For this review, take the finished solid that the model builds, in its own axes (mm). Face numbers are marked on the shaded views. A direction names the side the tool comes from. Give positions to 0.01 mm unless a question says otherwise; leave off trailing zeros. Order: outer loops, then holes, each group sorted by start corner. A loop starts at its lowest first (then second) coordinate and runs counter-clockwise, first axis right, second up. Notation, with made-up numbers: M 21,12 L 55,12 A16 cw 55,41 Z; hole C 7.5,22.25 d8. An arc over 180 degrees is marked long. Answer as CSV lines item,"result". Start each with the question number.
1. Clearance check with flat-ended pins moving along their axes: P1, Ø1.5, axis at x = -17.5, z = 0.5, coming from the +Y side; P2, Ø2.5, axis at x = -13.5, z = -18, coming from the -Y side; P3, Ø2.5, axis at y = 2.5, z = -16.5, coming from the -X side. State where each tip first meets the part, or that it passes through.
2. We need section B-B, the plane x = 0. Give the boundary of the cut face in (y, z), and give its area (3 significant figures).
3. Mouldability with a two-part tool opening along X and no side actions: class the marked faces 6, 7, 8 and 9 as pulls with the +X half, pulls with the -X half, needs draft (parallel to the pull), parting line crosses it, or undercut.
4. For line 1 along Z through (x, y) = (30, 14.25); line 2 along X through (y, z) = (6.75, -7.5); line 3 along X through (y, z) = (14.5, 16.5), list the stretches that pass through material, from the lowest coordinate up.
5. Machinability: for the marked faces 1, 2, 3, 4 and 5, which of the approach directions +Z, -Z, +X, -X, +Y, -Y give a long, thin tool a straight path to every point of the face, cutting with its end or side? Answer none if there is none.
6. We need section C-C, the plane z = 7.5. Give the boundary of the cut face in (x, y).
7. We need section A-A, the plane y = 15.5. State how many separate pieces and enclosed holes the cut face has, and give its area (3 significant figures).
8. We need section D-D, the plane x = 24. Give the boundary of the cut face in (y, z), and give its area (3 significant figures).
from build123d import *

# Parameters (mm, degrees)
SKETCH1_W                = 90
SKETCH1_H                = 30
BOSS_EXTRUDE1_DEPTH      = 7.5
SKETCH2_W                = 70
SKETCH2_H                = 30
BOSS_EXTRUDE2_DEPTH      = 10
CUT_EXTRUDE1_DEPTH       = 31
BOSS_EXTRUDE3_DEPTH      = 5
BOSS_EXTRUDE3_DEPTH_BACK = 35
CUT_EXTRUDE2_DEPTH       = 30
SKETCH7_R                = 2.25
CUT_EXTRUDE3_DEPTH       = 15


with BuildPart() as part:
    # Sketch1 → Boss-Extrude1 (new body, symmetric)
    with BuildSketch(Plane(origin=(0, 0, 0), x_dir=(1, 0, 0), z_dir=(0, 1, 0))):
        Rectangle(SKETCH1_W, SKETCH1_H)
    extrude(amount=BOSS_EXTRUDE1_DEPTH, both=True)

    # Sketch2 → Boss-Extrude2 (add)
    with BuildSketch(Plane(origin=(0, 7.5, 0), x_dir=(1, 0, 0), z_dir=(0, 1, 0))):
        Rectangle(SKETCH2_W, SKETCH2_H)
    extrude(amount=BOSS_EXTRUDE2_DEPTH)

    # Sketch3 → Cut-Extrude1 (cut, through all)
    with BuildSketch(Plane.XY.offset(15)):
        Polygon((-26.286782916, -2.5), (26.286782916, -2.5), (22.5, -7.5), (-22.5, -7.5), align=None)
    extrude(amount=-CUT_EXTRUDE1_DEPTH, mode=Mode.SUBTRACT)

    # Sketch4 → Boss-Extrude3 (add, two sides)
    with BuildSketch(Plane.XY.offset(15)) as boss_extrude3_sk:
        with BuildLine():
            Line((-7.5, 5), (-7.5, -2.5))
            Line((-7.5, -2.5), (7.5, -2.5))
            Line((7.5, -2.5), (7.5, 5))
            Line((7.5, 5), (17.5, 5))
            ThreePointArc((17.5, 5), (26.338834765, 8.661165235), (30, 17.5))
            Line((30, 17.5), (25, 17.5))
            ThreePointArc((25, 17.5), (17.5, 10), (10, 17.5))
            Line((10, 17.5), (-10, 17.5))
            ThreePointArc((-10, 17.5), (-17.5, 10), (-25, 17.5))
            Line((-25, 17.5), (-30, 17.5))
            ThreePointArc((-30, 17.5), (-26.338834765, 8.661165235), (-17.5, 5))
            Line((-17.5, 5), (-7.5, 5))
        make_face()
    extrude(amount=BOSS_EXTRUDE3_DEPTH)
    extrude(boss_extrude3_sk.sketch, amount=-BOSS_EXTRUDE3_DEPTH_BACK)

    # Sketch6 → Cut-Extrude2 (cut)
    with BuildSketch(Plane.XY.offset(15)):
        with BuildLine():
            Line((-25, 17.5), (-10, 17.5))
            ThreePointArc((-10, 17.5), (-17.5, 10), (-25, 17.5))
        make_face()
        with BuildLine():
            Line((10, 17.5), (25, 17.5))
            ThreePointArc((25, 17.5), (17.5, 10), (10, 17.5))
        make_face()
    extrude(amount=-CUT_EXTRUDE2_DEPTH, mode=Mode.SUBTRACT)

    # Sketch7 → Cut-Extrude3 (cut)
    with BuildSketch(Plane(origin=(0, 17.5, 0), x_dir=(1, 0, 0), z_dir=(0, 1, 0))):
        with Locations((0, 15)):
            Circle(SKETCH7_R)
        with Locations((0, -15)):
            Circle(SKETCH7_R)
        with Locations((-30, 7.5)):
            Circle(SKETCH7_R)
        with Locations((-30, -7.5)):
            Circle(SKETCH7_R)
        with Locations((30, -7.5)):
            Circle(SKETCH7_R)
        with Locations((30, 7.5)):
            Circle(SKETCH7_R)
    extrude(amount=-CUT_EXTRUDE3_DEPTH, mode=Mode.SUBTRACT)


solid = part.part
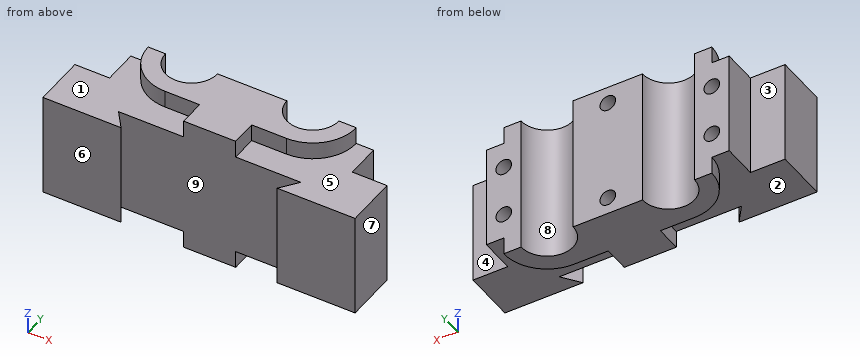
Result set:
1,P1,"y = 10.04"
1,P2,"y = 5"
1,P3,"x = -7.5"
2,outline,"M -2.5,-20 L 17.5,-20 L 17.5,-17.25 L 2.5,-17.25 L 2.5,-12.75 L 17.5,-12.75 L 17.5,12.75 L 2.5,12.75 L 2.5,17.25 L 17.5,17.25 L 17.5,20 L -2.5,20 Z"
2,area,"665 mm2"
3,face 6,"needs draft"
3,face 7,"pulls with the +X half"
3,face 8,"undercut"
3,face 9,"undercut"
4,line 1,"-15 to -9.75, -5.25 to 5.25, 9.75 to 15"
4,line 2,"-45 to -32.25, -27.75 to 27.75, 32.25 to 45"
4,line 3,"-29.63 to -24.37, -10.63 to -1.68, 1.68 to 10.63, 24.37 to 29.63"
5,face 1,"+Z, -X, -Y"
5,face 2,"-Z, -X, -Y"
5,face 3,"+Z, -Z, -X, +Y"
5,face 4,"+Z, -Z, +X, +Y"
5,face 5,"+Z, +X, -Y"
6,outline,"M -45,-7.5 L -22.5,-7.5 L -26.29,-2.5 L 26.29,-2.5 L 22.5,-7.5 L 45,-7.5 L 45,7.5 L 35,7.5 L 35,17.5 L 32.25,17.5 L 32.25,2.5 L 27.75,2.5 L 27.75,17.5 L 25,17.5 A7.5 cw 10,17.5 L -10,17.5 A7.5 cw -25,17.5 L -27.75,17.5 L -27.75,2.5 L -32.25,2.5 L -32.25,17.5 L -35,17.5 L -35,7.5 L -45,7.5 Z"
7,separate pieces,"3"
7,enclosed holes,"6"
7,area,"1,440 mm2"
8,outline,"M -7.5,-15 L -5.52,-15 L -5.52,15 L -7.5,15 Z; M -2.5,-15 L 6.82,-15 L 6.82,-20 L 13.76,-20 L 13.76,20 L 6.82,20 L 6.82,15 L -2.5,15 Z"
8,area,"617 mm2"
